Part model, mm, in its own coordinate system. A direction names the side the tool comes from. Round coordinates to 2 decimals unless told otherwise and drop trailing zeros. Write each loop counter-clockwise with the first axis right and the second up, starting at its lowest first coordinate (ties: lowest second). Pieces come first, ordered by that corner, then holes. Notation, with made-up numbers: (-15.5, 25.25) -> (22.5, 25.25) arc R27 cw to (22.5, 49.25) -> close; hole circle Ø11 at (-1.75, 69.25). An arc over 180 degrees is marked (long way). Return JSON: item names as keys, results as strings. Group by question number.
(1) Saw through at A-A (x = 0). List the corners of the cut face in (y, z).
(2) Mould opens along X. For faces 4 (the flat face through (-12.7, 2, 69)), 5 (the cylindrical face through (-17.8, 2, 17.9)), 6 (the flat face through (-13, -18.288, -1)), 7 (the flat face through (12.7, 2, -69)) say: +X half, -X half, draft (parallel to the pull), parting line (faces both ways), or undercut.
(3) Drop flat-ended pins along their axis: pin 1 Ø9 at (y, z) = (-6, -6) entering from -X; pin 2 Ø6.5 at (y, z) = (-10.033, -34.417) entering from +X; pin 3 Ø4.5 at (x, z) = (-19.05, -19.05) entering from -Y. Give the stop position or say it passes through.
(4) Tool access for faces 1 (the flat face through (13, -9, 44.45)), 2 (the flat face through (-13, -9, -44.45)), 3 (the flat face through (-15.16, -9, 1)): list every direction of +Z, -Z, +X, -X, +Y, -Y with a clear straight run to the whole face (end or side of a thin tool).
(5) Saw through at D-D (z = 19.05). List the corners of the cut face in (x, y).
(6) Saw through at B-B (y = -3.5). List the corners of the cut face in (x, z), plus the area to 3 significant figures.
(7) Drill centre lines: L1, parallel to Z at x = 0, y = 2.8; L2, parallel to X at y = -2, z = 40.5; L3, parallel to X at y = 1.2, z = -81.28. Where is each one in solid material? Low to high. Write a range as from..to.
(8) Saw through at C-C (z = 81.28). List the corners of the cut face in (x, y).
from build123d import *

# Parameters (mm, degrees)
BOSS_EXTRUDE1_DEPTH  = 4
SKETCH3_W            = 5
SKETCH3_H            = 88.9
BOSS_EXTRUDE2_DEPTH  = 18.288
M3_CLEARANCE_HOLE1_D = 3.4
FILLET1_R            = 0.5
SKETCH6_R            = 2.54
CUT_EXTRUDE1_DEPTH   = 66.96
SKETCH7_R            = 2.54
CUT_EXTRUDE2_DEPTH   = 23.288


with BuildPart() as part:
    # Sketch1 → Boss-Extrude1 (new body)
    with BuildSketch(Plane(origin=(0, 0, 0), x_dir=(1, 0, 0), z_dir=(0, 1, 0))):
        with BuildLine():
            Line((-12.7, 49.186888497), (-12.7, 88.9))
            Line((-12.7, 88.9), (12.7, 88.9))
            Line((12.7, 88.9), (12.7, 49.186888497))
            ThreePointArc((12.7, 49.186888497), (50.8, 0), (12.7, -49.186888497))
            Line((12.7, -49.186888497), (12.7, -88.9))
            Line((12.7, -88.9), (-12.7, -88.9))
            Line((-12.7, -88.9), (-12.7, -49.186888497))
            ThreePointArc((-12.7, -49.186888497), (-50.8, 0), (-12.7, 49.186888497))
        make_face()
    extrude(amount=BOSS_EXTRUDE1_DEPTH)

    # Sketch3 → Boss-Extrude2 (add)
    with BuildSketch(Plane(origin=(0, 0, 0), x_dir=(-1, 0, 0), z_dir=(0, -1, 0))):
        with Locations((12.66, 0)):
            Rectangle(SKETCH3_W, SKETCH3_H)
        with Locations((-12.66, 0)):
            Rectangle(SKETCH3_W, SKETCH3_H)
    extrude(amount=BOSS_EXTRUDE2_DEPTH)

    # M3 Clearance Hole1 (through all)
    with Locations(Plane(origin=(0, 4, 0), x_dir=(1, 0, 0), z_dir=(0, 1, 0))):
        with Locations((-19.05, -19.05), (19.05, -19.05), (-19.05, 19.05), (19.05, 19.05)):
            Hole(M3_CLEARANCE_HOLE1_D / 2)

    # Fillet1
    fillet1_edges = [part.edges().sort_by_distance(p)[0] for p in [
        (-15.16, 0, 0),
        (-12.66, 0, -44.45),
        (-12.66, 0, 44.45),
        (12.66, 0, -44.45),
        (15.16, 0, 0),
        (12.66, 0, 44.45),
    ]]
    fillet(fillet1_edges, radius=FILLET1_R)

    # Sketch6 → Cut-Extrude1 (cut, through all)
    with BuildSketch(Plane.ZY.offset(15.16)):
        with Locations((34.417, -10.033)):
            Circle(SKETCH6_R)
        with Locations((-34.417, -10.033)):
            Circle(SKETCH6_R)
    extrude(amount=-CUT_EXTRUDE1_DEPTH, mode=Mode.SUBTRACT)

    # Sketch7 → Cut-Extrude2 (cut, through all)
    with BuildSketch(Plane(origin=(0, 4, 0), x_dir=(1, 0, 0), z_dir=(0, 1, 0))):
        with Locations((0, 81.28)):
            Circle(SKETCH7_R)
        with Locations((0, -81.28)):
            Circle(SKETCH7_R)
    extrude(amount=-CUT_EXTRUDE2_DEPTH, mode=Mode.SUBTRACT)


solid = part.part
Computed values:
{
 "1": {"outline": "(0, -88.9) -> (4, -88.9) -> (4, -83.82) -> (0, -83.82) -> close; (0, -78.74) -> (4, -78.74) -> (4, 78.74) -> (0, 78.74) -> close; (0, 83.82) -> (4, 83.82) -> (4, 88.9) -> (0, 88.9) -> close"},
 "2": {"face 4": "-X half", "face 5": "undercut", "face 6": "draft", "face 7": "+X half"},
 "3": {"pin 1": "x = -15.16", "pin 2": "x = 15.16", "pin 3": "y = 0"},
 "4": {"face 1": "+Z, +X, -X, -Y", "face 2": "-Z, +X, -X, -Y", "face 3": "+Z, -Z, -X, -Y"},
 "5": {"outline": "(-47.09, 0) -> (-20.75, 0) -> (-20.75, 4) -> (-47.09, 4) -> close; (-17.35, 0) -> (-15.66, 0) arc R0.5 cw to (-15.16, -0.5) -> (-15.16, -18.29) -> (-10.16, -18.29) -> (-10.16, 0) -> (10.16, 0) -> (10.16, -18.29) -> (15.16, -18.29) -> (15.16, -0.5) arc R0.5 cw to (15.66, 0) -> (17.35, 0) -> (17.35, 4) -> (-17.35, 4) -> close; (20.75, 0) -> (47.09, 0) -> (47.09, 4) -> (20.75, 4) -> close"},
 "6": {"outline": "(-15.16, -44.45) -> (-10.16, -44.45) -> (-10.16, 44.45) -> (-15.16, 44.45) -> close; (10.16, -44.45) -> (15.16, -44.45) -> (15.16, 44.45) -> (10.16, 44.45) -> close", "area": "889 mm2"},
 "7": {"L1": "-88.9..-83.82, -78.74..78.74, 83.82..88.9", "L2": "-15.16..-10.16, 10.16..15.16", "L3": "-12.7..-2.54, 2.54..12.7"},
 "8": {"outline": "(-12.7, 0) -> (-2.54, 0) -> (-2.54, 4) -> (-12.7, 4) -> close; (2.54, 0) -> (12.7, 0) -> (12.7, 4) -> (2.54, 4) -> close"}
}
